Check sheet for the modelled part. Datum: model origin and axes. Units: mm. A direction names the side the tool comes from. Coordinates: 2 decimals unless noted, no trailing zeros. Loops run counter-clockwise (first coordinate to the right, second up) from the corner with the lowest first, then second, coordinate; pieces in that order, holes last. Notation, with made-up numbers: M 46,83 L 69,83 A20 cw 69,111 Z; hole C 40.5,66.5 d6. An arc over 180 degrees is marked long. Return JSON: item names as keys, results as strings.
from build123d import *

# Parameters (mm, degrees)
SKETCH_1_R      = 5.0225
SKETCH_1_R_2    = 2.05
EXTRUDE_1_DEPTH = 3
FILLET_1_R      = 2
FILLET_2_R      = 1.3
SKETCH_3_R      = 5.025
EXTRUDE_2_DEPTH = 3


with BuildPart() as part:
    # 草图1 → 凸台-拉伸1 (new body)
    with BuildSketch(Plane.XY):
        with BuildLine():
            Line((298.545628784, -83.894391363), (298.545628784, -92.841778663))
            Line((298.545628784, -92.841778663), (302.545628784, -92.841778663))
            Line((302.545628784, -92.841778663), (302.545628784, -91.391778663))
            Line((302.545628784, -91.391778663), (305.745628784, -91.391778663))
            Line((305.745628784, -91.391778663), (305.745628784, -92.841778663))
            Line((305.745628784, -92.841778663), (308.945628784, -92.841778663))
            Line((308.945628784, -92.841778663), (308.945628784, -96.941778663))
            Line((308.945628784, -96.941778663), (305.745628784, -96.941778663))
            Line((305.745628784, -96.941778663), (305.745628784, -98.391778663))
            Line((305.745628784, -98.391778663), (302.545628784, -98.391778663))
            Line((302.545628784, -98.391778663), (302.545628784, -96.941778663))
            Line((302.545628784, -96.941778663), (298.545628784, -96.941778663))
            Line((298.545628784, -96.941778663), (298.545628784, -105.894391358))
            Line((298.545628784, -105.894391358), (293.545628784, -105.894391358))
            Line((293.545628784, -105.894391358), (293.545628784, -113.894391358))
            Line((293.545628784, -113.894391358), (298.545628784, -113.894391358))
            Line((298.545628784, -113.894391358), (298.545628784, -122.847004054))
            Line((298.545628784, -122.847004054), (302.545628784, -122.847004054))
            Line((302.545628784, -122.847004054), (302.545628784, -121.397004054))
            Line((302.545628784, -121.397004054), (305.745628784, -121.397004054))
            Line((305.745628784, -121.397004054), (305.745628784, -122.847004054))
            Line((305.745628784, -122.847004054), (308.945628784, -122.847004054))
            Line((308.945628784, -122.847004054), (308.945628784, -126.947004054))
            Line((308.945628784, -126.947004054), (305.745628784, -126.947004054))
            Line((305.745628784, -126.947004054), (305.745628784, -128.397004054))
            Line((305.745628784, -128.397004054), (302.545628784, -128.397004054))
            Line((302.545628784, -128.397004054), (302.545628784, -126.947004054))
            Line((302.545628784, -126.947004054), (298.545628784, -126.947004054))
            Line((298.545628784, -126.947004054), (298.545628784, -140.447004054))
            Line((298.545628784, -140.447004054), (324.188862368, -140.447004054))
            Line((324.188862368, -140.447004054), (376.358604426, -71.946984141))
            Line((376.358604426, -71.946984141), (376.358604426, 4.396201153))
            ThreePointArc((376.358604426, 4.396201153), (348.536987634, 32.217817945), (320.715370843, 4.396201153))
            Line((320.715370843, 4.396201153), (307.936987634, -35.346984141))
            Line((307.936987634, -35.346984141), (298.545628784, -35.346984141))
            Line((298.545628784, -35.346984141), (298.545628784, -45.889165972))
            Line((298.545628784, -45.889165972), (293.545628784, -45.889165972))
            Line((293.545628784, -45.889165972), (293.545628784, -53.889165972))
            Line((293.545628784, -53.889165972), (298.545628784, -53.889165972))
            Line((298.545628784, -53.889165972), (298.545628784, -62.841778668))
            Line((298.545628784, -62.841778668), (302.545628784, -62.841778668))
            Line((302.545628784, -62.841778668), (302.545628784, -61.391778668))
            Line((302.545628784, -61.391778668), (305.745628784, -61.391778668))
            Line((305.745628784, -61.391778668), (305.745628784, -62.841778668))
            Line((305.745628784, -62.841778668), (308.945628784, -62.841778668))
            Line((308.945628784, -62.841778668), (308.945628784, -66.941778668))
            Line((308.945628784, -66.941778668), (305.745628784, -66.941778668))
            Line((305.745628784, -66.941778668), (305.745628784, -68.391778668))
            Line((305.745628784, -68.391778668), (302.545628784, -68.391778668))
            Line((302.545628784, -68.391778668), (302.545628784, -66.941778668))
            Line((302.545628784, -66.941778668), (298.545628784, -66.941778668))
            Line((298.545628784, -66.941778668), (298.545628784, -75.894391363))
            Line((298.545628784, -75.894391363), (293.545628784, -75.894391363))
            Line((293.545628784, -75.894391363), (293.545628784, -83.894391363))
            Line((293.545628784, -83.894391363), (298.545628784, -83.894391363))
        make_face()
        with Locations((348.536987634, 4.396201153)):
            Circle(SKETCH_1_R, mode=Mode.SUBTRACT)
        with Locations((320.545628784, -134.447004054)):
            Circle(SKETCH_1_R_2, mode=Mode.SUBTRACT)
        with Locations((370.358604426, -65.946984141)):
            Circle(SKETCH_1_R_2, mode=Mode.SUBTRACT)
        with Locations((313.936987634, -41.346984141)):
            Circle(SKETCH_1_R_2, mode=Mode.SUBTRACT)
        Polygon((354.947285032, -70.136765586), (328.579617375, -106.396108383), (325.08144343, -57.115165973), align=None, mode=Mode.SUBTRACT)
        Polygon((329.571126451, -37.254352656), (354.337315751, -48.052488042), (344.758747766, -17.175445836), align=None, mode=Mode.SUBTRACT)
    extrude(amount=EXTRUDE_1_DEPTH)

    # 圆角1
    fillet_1_edges = [part.edges().sort_by_distance(p)[0] for p in [
        (354.947285032, -70.136765586, 1.5),
        (325.08144343, -57.115165973, 1.5),
        (328.579617375, -106.396108383, 1.5),
        (344.758747766, -17.175445836, 1.5),
        (329.571126451, -37.254352656, 1.5),
        (354.337315751, -48.052488042, 1.5),
    ]]
    fillet(fillet_1_edges, radius=FILLET_1_R)

    # 圆角2
    fillet_2_edges = [part.edges().sort_by_distance(p)[0] for p in [
        (293.545628784, -113.894391358, 1.5),
        (293.545628784, -105.894391358, 1.5),
        (293.545628784, -83.894391363, 1.5),
        (293.545628784, -75.894391363, 1.5),
        (293.545628784, -53.889165972, 1.5),
        (293.545628784, -45.889165972, 1.5),
    ]]
    fillet(fillet_2_edges, radius=FILLET_2_R)

    # 草图3 → 凸台-拉伸2 (add)
    with BuildSketch(Plane(origin=(0, 0, 0), x_dir=(-1, 0, 0), z_dir=(0, 0, -1))):
        with BuildLine():
            Line((-348.536987634, 28.396201153), (-396.833278949, 30.337153408))
            ThreePointArc((-396.833278949, 30.337153408), (-409.833278949, 17.337153408), (-396.833278949, 4.337153408))
            Line((-396.833278949, 4.337153408), (-348.536987634, -19.603798847))
            Line((-348.536987634, -19.603798847), (-372.536987634, 4.396201153))
            Line((-372.536987634, 4.396201153), (-348.536987634, 28.396201153))
        make_face()
        with Locations((-396.833278949, 17.337153408)):
            Circle(SKETCH_3_R, mode=Mode.SUBTRACT)
    extrude(amount=-EXTRUDE_2_DEPTH)


solid = part.part
1) Section check C-C on z = 1.75. Count the separate pieces of the cut face and the enclosed holes in it, then the cut area to 3 significant figures.
Answers:
{"separate pieces": "1", "enclosed holes": "7", "area": "9,810 mm²"}
2) Draft check along X on faces 1 (the face through (386.739, -0.667, 1.479)), 2 (the face through (340.215, -63.713, 1.479)), 3 (the face through (338, -53, 0)). Enter one of: +X half, -X half, draft (parallel to the pull), parting line (faces both ways), or undercut.
Answers:
{"face 1": "+X half", "face 2": "undercut", "face 3": "draft"}
3) Scan lines: line 1 along Y through (x, z) = (305.5, 1.8); line 2 along Y through (x, z) = (299, 1.1); line 3 along Y through (x, z) = (335, 1.75). Record each from-to range of solid material in increasing order. Write a range as [from, to].
Answers:
{"line 1": "[-140.45, -128.4], [-121.4, -98.39], [-91.39, -68.39], [-61.39, -35.35]", "line 2": "[-140.45, -126.95], [-122.85, -96.94], [-92.84, -66.94], [-62.84, -35.35]", "line 3": "[-126.25, -97.57], [-61.44, -39.62], [-30.08, 28.7]"}
4) Section check D-D on x = 379. Record the cut outline in (y, z), then the cut area to 3 significant figures.
Answers:
{"outline": "M -4.5,0 L 29.62,0 L 29.62,3 L -4.5,3 Z", "area": "102 mm²"}
5) Section check A-A on y = -80.5. Record the cut outline in (x, z), then the cut area to 3 significant figures.
Answers:
{"outline": "M 293.55,0 L 326.74,0 L 326.74,3 L 293.55,3 Z; M 347.41,0 L 369.84,0 L 369.84,3 L 347.41,3 Z", "area": "167 mm²"}
6) Section check B-B on y = -49. Record the cut outline in (x, z).
Answers:
{"outline": "M 293.55,0 L 376.36,0 L 376.36,3 L 293.55,3 Z"}
7) Set-up check for faces 4 (the face through (336.8, -27.7, 1.5)), 5 (the face through (334.59, 28.47, 1.48)): record each of +Z, -Z, +X, -X, +Y, -Y from which the full face is reachable in a straight line by a thin tool's end or side.
Answers:
{"face 4": "+Z, -Z", "face 5": "+Z, -Z, +Y"}
8) Go/stop test with flat-tipped pins: pin 1 Ø1.5 at (y, z) = (-125, 2) entering from -X; pin 2 Ø1 at (y, z) = (-41, 2) entering from +X; pin 3 Ø6 at (x, y) = (359, -101.5) entering from +Z; pin 4 Ø0.9 at (y, z) = (-60, 1.5) entering from -X. Record where each tip stops, or that it passes through.
Answers:
{"pin 1": "x = 308.95", "pin 2": "x = 376.36", "pin 3": "through", "pin 4": "x = 298.55"}
